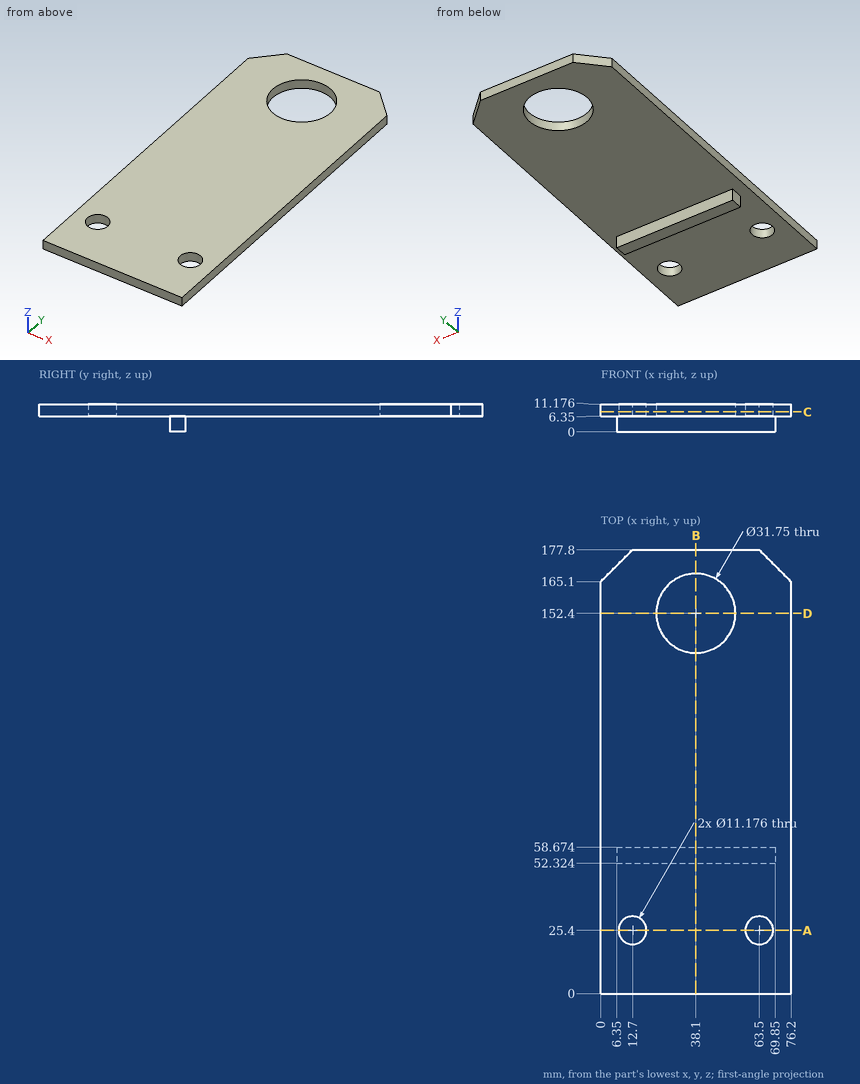
Job drawing, mm, ordinate dimensions from the low corner. One solid piece. Coordinates: 2 decimals unless noted, no trailing zeros. Write each loop counter-clockwise with the first axis right and the second up, starting at its lowest first coordinate (ties: lowest second). Pieces come first, ordered by that corner, then holes. Notation, with made-up numbers: (-11.5, 5.5) - (-5.5, 5.5) arc R25 cw to (-5.5, 28.5) - close; hole circle Ø5 at (44.25, -13.75). An arc over 180 degrees is marked (long way). Use a Markdown table: item, result. Add a question column.
Item 1: Band-saw the part on B-B, the plane x = 38.1. Give the cut face in (y, z) (3 decimals).
Item 2: Flat gauge pins, fed straight in: pin 1 (3 mm diameter, centred on x = 45, z = 4, fed in from -Y); pin 2 (3 mm diameter, centred on x = 29, y = 123, fed in from -Z); pin 3 (4 mm diameter, centred on x = 68, z = 9.5, fed in from +Y). Where does each tip first touch, or does it go through?
Item 3: Band-saw the part on D-D, the plane y = 152.4. Give the cut face in (x, z) (3 decimals), and give its area (3 significant figures).
Item 4: Band-saw the part on C-C, the plane z = 8. Give the cut face in (x, y) (3 decimals).
Item 5: Band-saw the part on A-A, the plane y = 25.4. Give the cut face in (x, z).
Item 6: Drill centre lines: L1, parallel to Y at x = 38.1, z = 8.5 (3 decimals); L2, parallel to Y at x = 12.7, z = 9.5; L3, parallel to Z at x = 6, y = 48. Where is each one in solid material? Low to high. Write a range as from..to.
Numbers:
| question | item | result |
|---|---|---|
| 1 | outline | (0, 6.35) - (52.324, 6.35) - (52.324, 0) - (58.674, 0) - (58.674, 6.35) - (136.525, 6.35) - (136.525, 11.176) - (0, 11.176) - close; (168.275, 6.35) - (177.8, 6.35) - (177.8, 11.176) - (168.275, 11.176) - close |
| 2 | pin 1 | y = 52.32 |
| 2 | pin 2 | z = 6.35 |
| 2 | pin 3 | y = 175.3 |
| 3 | outline | (0, 6.35) - (22.225, 6.35) - (22.225, 11.176) - (0, 11.176) - close; (53.975, 6.35) - (76.2, 6.35) - (76.2, 11.176) - (53.975, 11.176) - close |
| 3 | area | 215 mm2 |
| 4 | outline | (0, 0) - (76.2, 0) - (76.2, 165.1) - (63.5, 177.8) - (12.7, 177.8) - (0, 165.1) - close; hole circle Ø11.176 at (12.7, 25.4); hole circle Ø31.75 at (38.1, 152.4); hole circle Ø11.176 at (63.5, 25.4) |
| 5 | outline | (0, 6.35) - (7.11, 6.35) - (7.11, 11.18) - (0, 11.18) - close; (18.29, 6.35) - (57.91, 6.35) - (57.91, 11.18) - (18.29, 11.18) - close; (69.09, 6.35) - (76.2, 6.35) - (76.2, 11.18) - (69.09, 11.18) - close |
| 6 | L1 | 0..136.525, 168.275..177.8 |
| 6 | L2 | 0..19.81, 30.99..177.8 |
| 6 | L3 | 6.35..11.18 |
